Geometry: final body of the model. Coordinates: model frame, mm. A direction names the side the tool comes from. Coordinates: 2 decimals unless noted, no trailing zeros. Write each loop counter-clockwise with the first axis right and the second up, starting at its lowest first coordinate (ties: lowest second). Pieces come first, ordered by that corner, then holes. Notation, with made-up numbers: (-19, -23) -> (32, -23) arc R27 ccw to (32, 12) -> close; hole circle Ø2 at (17, -32.75). An arc over 180 degrees is marked (long way). One line per item, written item: value.
```python
from build123d import *

# Parameters (mm, degrees)
BASPROSKE_W         = 12.5
BASPROSKE_H         = 18.75
TOOTHCUT_DEPTH      = 30.315098499
TEETHCUTS_COUNT     = 28
TEETHCUTS_ANGLE     = 347.142857143
BORSKE_R            = 1
BORE_DEPTH          = 50.0000508
CUT_EXTRUDE1_DEPTH  = 30.212056464
SKETCH2_R           = 3.28
BOSS_EXTRUDE1_DEPTH = 1.5


with BuildPart() as part:
    # BasProSke → Base-Revolve (revolve)
    with BuildSketch(Plane(origin=(0, 0, 0), x_dir=(1, 0, 0), z_dir=(0, 1, 0)), mode=Mode.PRIVATE) as base_revolve_sk:
        with Locations((6.25, 9.375)):
            Rectangle(BASPROSKE_W, BASPROSKE_H)
    revolve(base_revolve_sk.sketch.rotate(Axis((-10, 0, 0), (1, 0, 0)), 180), axis=Axis((-10, 0, 0), (1, 0, 0)))

    # TooCutSke → ToothCut (cut, through all)
    with BuildSketch(Plane(origin=(0, 0, 0), x_dir=(0, 0, -1), z_dir=(1, 0, 0))):
        with BuildLine():
            ThreePointArc((0.585229427, 15.925750807), (0, 15.9365), (-0.585229427, 15.925750807))
            ThreePointArc((-0.585229427, 15.925750807), (-1.019072842, 17.372951322), (-1.753340618, 18.693352878))
            ThreePointArc((-1.753340618, 18.693352878), (0, 18.7754), (1.753340618, 18.693352878))
            ThreePointArc((1.753340618, 18.693352878), (1.019072842, 17.372951322), (0.585229427, 15.925750807))
        make_face()
    toothcut = extrude(amount=TOOTHCUT_DEPTH, mode=Mode.SUBTRACT)

    # TeethCuts: ToothCut ×28 about axis
    teethcuts_axis = Axis((-10, 0, 0), (1, 0, 0))
    for i in range(1, TEETHCUTS_COUNT):
        add(toothcut.rotate(teethcuts_axis, i * TEETHCUTS_ANGLE / (TEETHCUTS_COUNT - 1)), mode=Mode.SUBTRACT)

    # BorSke → Bore (cut, symmetric)
    with BuildSketch(Plane(origin=(0, 0, 0), x_dir=(0, 0, -1), z_dir=(1, 0, 0))):
        with Locations(Location((0, 0, 0), (0, 0, 180))):
            Circle(BORSKE_R)
    extrude(amount=BORE_DEPTH, both=True, mode=Mode.SUBTRACT)

    # Sketch1 → Cut-Extrude1 (cut, through all)
    with BuildSketch(Plane.ZY):
        with BuildLine():
            Line((-2.88, 1.56971335), (-2.88, -1.56971335))
            ThreePointArc((-2.88, -1.56971335), (3.28, 0), (-2.88, 1.56971335))
        make_face()
    extrude(amount=-CUT_EXTRUDE1_DEPTH, mode=Mode.SUBTRACT)

    # Sketch2 → Boss-Extrude1 (add)
    with BuildSketch(Plane.ZY):
        Circle(SKETCH2_R)
    extrude(amount=-BOSS_EXTRUDE1_DEPTH)


solid = part.part
```
(1) Section B-B (y = 0). Return the cut outline in (x, z), then the cut area to 3 significant figures.
Responses:
outline: (0, -15.94) -> (12.5, -15.94) -> (12.5, -2.88) -> (1.5, -2.88) -> (1.5, 3.28) -> (12.5, 3.28) -> (12.5, 15.94) -> (0, 15.94) -> close
area: 331 mm2
(2) First-contact query: pin 1 (4 mm diameter, centred on x = 6, z = 10.5, fed in from -Y); pin 2 (1.8 mm diameter, centred on y = 1, z = 1.5, fed in from +X); pin 3 (1.5 mm diameter, centred on x = 9.5, z = -0.5, fed in from +Y). Flat tips, straight axial feed; report the tip coordinate or a pass-through.
Responses:
pin 1: stops at y = -16.07
pin 2: stops at x = 1.5
pin 3: stops at y = 17.87
(3) Reachability of faces 1 (the cylindrical face through (6.162, -16.716, 4.863)), 2 (the cylindrical face through (6.162, -6.618, -16.059)), 3 (the cylindrical face through (6.162, 16.682, 4.839)), 4 (the cylindrical face through (6.923, -0.121, 3.278)), 5 (the cylindrical face through (6.162, 8.429, -15.187)) from +Z, -Z, +X, -X, +Y, -Y: full face, straight path, thin tool, end or side. Return the list, or none.
Responses:
face 1: +X, -X, -Y
face 2: +X, -X
face 3: +X, -X, +Y
face 4: +X
face 5: -Z, +X, -X
(4) Pull-direction query (Z, two-part tool) for faces 6 (the cylindrical face through (6.16, 1.02, 17.38)), 7 (the cylindrical face through (6.162, -0.008, -15.936)), 8 (the cylindrical face through (6.162, 9.943, 12.455)); classes: released by +Z, released by -Z, zero draft, split by the parting line, or undercut.
Responses:
face 6: released by +Z
face 7: released by -Z
face 8: undercut
(5) Section A-A (z = 0). Return the cut outline in (x, y).
Responses:
outline: (0, -15.94) -> (12.5, -15.94) -> (12.5, -3.28) -> (1.5, -3.28) -> (1.5, 3.28) -> (12.5, 3.28) -> (12.5, 15.94) -> (0, 15.94) -> close
(6) Line query: line 1 (Y direction, x = 6, z = 0); line 2 (Z direction, x = 9.75, y = 0); line 3 (Z direction, x = 7.75, y = 17). Output: solid intervals per line, ascending. Write a range as [from, to].
Responses:
line 1: y = [-15.94, -3.28], [3.28, 15.94]
line 2: z = [-15.94, -2.88], [3.28, 15.94]
line 3: z = [-6.61, -5.08], [-2.9, -0.87], [0.87, 2.9], [5.08, 6.61]
